```python
from build123d import *

# Parameters (mm, degrees)
F1_DEPTH  = 15.875
F3_DEPTH  = 15.876
F4_R      = 15.1511
F5_DEPTH  = 15.876
F6_R      = 57.277
F7_DEPTH  = 6.35
F8_R      = 4.953
F9_DEPTH  = 15.876
F11_DEPTH = 9.525
F13_R     = 5.4864
F14_DEPTH = 15.875
F16_DEPTH = 1.27


with BuildPart() as f1:
    # F0 (on Top) → F1 (new body)
    with BuildSketch(Plane.XY):
        with BuildLine():
            Line((261.564905, -58.477244), (113.604486, -6.008632))
            ThreePointArc((113.604486, -6.008632), (0, -82.6643), (113.604486, -159.319968))
            Line((113.604486, -159.319968), (261.564905, -106.851356))
            Line((261.564905, -106.851356), (263.024603, -106.333729))
            ThreePointArc((263.024603, -106.333729), (279.2095, -82.6643), (263.024603, -58.994871))
            Line((263.024603, -58.994871), (261.564905, -58.477244))
        make_face()
        with BuildLine():
            ThreePointArc((263.024603, -58.994871), (262.2987, -58.724929), (261.564905, -58.477244))
            Line((261.564905, -58.477244), (263.024603, -58.994871))
        make_face()
        with BuildLine():
            Line((263.024603, -106.333729), (261.564905, -106.851356))
            ThreePointArc((261.564905, -106.851356), (262.2987, -106.603671), (263.024603, -106.333729))
        make_face()
    extrude(amount=F1_DEPTH)

    # F2 (on face) → F3 (cut, through all)
    with BuildSketch(Plane.XY.offset(15.875)):
        with BuildLine():
            ThreePointArc((266.5095, -82.6643), (253.8095, -69.9643), (241.1095, -82.6643))
            Line((241.1095, -82.6643), (266.5095, -82.6643))
        make_face()
        with BuildLine():
            Line((266.5095, -82.6643), (241.1095, -82.6643))
            ThreePointArc((241.1095, -82.6643), (253.8095, -95.3643), (266.5095, -82.6643))
        make_face()
    extrude(amount=-F3_DEPTH, mode=Mode.SUBTRACT)

    # F4 (on face) → F5 (cut, through all)
    with BuildSketch(Plane.XY.offset(15.875)):
        with Locations((82.3595, -82.6643)):
            Circle(F4_R)
    extrude(amount=-F5_DEPTH, mode=Mode.SUBTRACT)

    # F6 (on face) → F7 (cut)
    with BuildSketch(Plane(origin=(0, 0, 0), x_dir=(1, 0, 0), z_dir=(0, 0, -1))):
        with Locations((82.3595, 82.6643)):
            Circle(F6_R)
    extrude(amount=-F7_DEPTH, mode=Mode.SUBTRACT)

    # F8 (on face) → F9 (cut, through all)
    with BuildSketch(Plane(origin=(0, 0, 0), x_dir=(1, 0, 0), z_dir=(0, 0, -1))):
        with Locations((29.6545, 135.3693)):
            Circle(F8_R)
        with Locations((135.0645, 135.3693)):
            Circle(F8_R)
        with Locations((135.0645, 29.9593)):
            Circle(F8_R)
        with Locations((29.6545, 29.9593)):
            Circle(F8_R)
    extrude(amount=-F9_DEPTH, mode=Mode.SUBTRACT)

    # F10 (on face) → F11 (cut)
    with BuildSketch(Plane(origin=(0, 0, 0), x_dir=(1, 0, 0), z_dir=(0, 0, -1))):
        with BuildLine():
            ThreePointArc((57.15, 82.6643), (56.220064, 84.909364), (53.975, 85.8393))
            Line((53.975, 85.8393), (0.060996, 85.8393))
            Line((0.060996, 85.8393), (-2.488084, 85.8393))
            Line((-2.488084, 85.8393), (-2.488084, 79.4893))
            Line((-2.488084, 79.4893), (-1.513804, 79.4893))
            Line((-1.513804, 79.4893), (53.975, 79.4893))
            ThreePointArc((53.975, 79.4893), (56.220064, 80.419236), (57.15, 82.6643))
        make_face()
    extrude(amount=-F11_DEPTH, mode=Mode.SUBTRACT)

    # F13 (on offset) → F14 (cut)
    with BuildSketch(Plane.YZ.offset(279.4)):
        with Locations((-82.6643, 7.9375)):
            Circle(F13_R)
    extrude(amount=-F14_DEPTH, mode=Mode.SUBTRACT)

    # F15 (on face) → F16 (cut)
    with BuildSketch(Plane.XY.offset(15.875)):
        with BuildLine():
            Line((167.299575, -48.660433), (144.385987, -48.660433))
            Line((144.385987, -48.660433), (148.052161, -55.010433))
            Line((148.052161, -55.010433), (172.798837, -55.010433))
            ThreePointArc((172.798837, -55.010433), (173.592587, -55.223117), (174.173652, -55.804183))
            Line((174.173652, -55.804183), (207.672688, -113.826216))
            Line((207.672688, -113.826216), (214.81237, -113.492506))
            Line((214.81237, -113.492506), (172.90237, -40.902257))
            Line((172.90237, -40.902257), (165.468663, -40.726699))
            Line((165.468663, -40.726699), (168.674391, -46.279183))
            ThreePointArc((168.674391, -46.279183), (168.674391, -47.866683), (167.299575, -48.660433))
        make_face()
        with BuildLine():
            Line((165.826053, -66.122933), (171.684878, -66.122933))
            Line((171.684878, -66.122933), (175.980346, -73.562901))
            Line((175.980346, -73.562901), (177.355162, -72.769151))
            Line((177.355162, -72.769151), (178.729977, -71.975401))
            Line((178.729977, -71.975401), (174.434509, -64.535433))
            ThreePointArc((174.434509, -64.535433), (173.272378, -63.373302), (171.684878, -62.947933))
            Line((171.684878, -62.947933), (156.301053, -62.947933))
            ThreePointArc((156.301053, -62.947933), (153.551422, -64.535433), (153.551422, -67.710433))
            Line((153.551422, -67.710433), (156.930346, -73.562901))
            Line((156.930346, -73.562901), (158.305162, -72.769151))
            Line((158.305162, -72.769151), (159.679977, -71.975401))
            Line((159.679977, -71.975401), (156.301053, -66.122933))
            Line((156.301053, -66.122933), (162.159878, -66.122933))
            Line((162.159878, -66.122933), (165.095358, -71.207332))
            Line((165.095358, -71.207332), (167.844988, -69.619832))
            Line((167.844988, -69.619832), (165.826053, -66.122933))
        make_face()
        with BuildLine():
            Line((166.832487, -84.363913), (162.863737, -77.489836))
            Line((162.863737, -77.489836), (160.114107, -79.077336))
            Line((160.114107, -79.077336), (164.082857, -85.951413))
            ThreePointArc((164.082857, -85.951413), (166.010737, -87.430727), (168.419987, -87.113543))
            Line((168.419987, -87.113543), (179.957857, -80.452151))
            Line((179.957857, -80.452151), (183.926607, -87.326228))
            Line((183.926607, -87.326228), (186.676237, -85.738728))
            Line((186.676237, -85.738728), (182.707487, -78.864651))
            ThreePointArc((182.707487, -78.864651), (180.779607, -77.385337), (178.370357, -77.702521))
            Line((178.370357, -77.702521), (166.832487, -84.363913))
        make_face()
        with BuildLine():
            Line((172.176053, -93.619239), (187.559878, -93.619239))
            Line((187.559878, -93.619239), (191.864107, -101.074381))
            Line((191.864107, -101.074381), (194.613737, -99.486881))
            Line((194.613737, -99.486881), (190.309509, -92.031739))
            ThreePointArc((190.309509, -92.031739), (189.147378, -90.869609), (187.559878, -90.444239))
            Line((187.559878, -90.444239), (172.176053, -90.444239))
            ThreePointArc((172.176053, -90.444239), (169.426422, -92.031739), (169.426422, -95.206739))
            Line((169.426422, -95.206739), (172.814107, -101.074381))
            Line((172.814107, -101.074381), (175.563737, -99.486881))
            Line((175.563737, -99.486881), (172.176053, -93.619239))
        make_face()
        with BuildLine():
            Line((201.252318, -110.681192), (198.234108, -105.717761))
            ThreePointArc((198.234108, -105.717761), (197.077421, -104.599884), (195.521297, -104.192393))
            Line((195.521297, -104.192393), (180.187231, -104.192393))
            ThreePointArc((180.187231, -104.192393), (177.419723, -105.811268), (177.474421, -109.017024))
            Line((177.474421, -109.017024), (180.492631, -113.980455))
            ThreePointArc((180.492631, -113.980455), (181.649318, -115.098332), (183.205442, -115.505824))
            Line((183.205442, -115.505824), (198.539508, -115.505824))
            ThreePointArc((198.539508, -115.505824), (201.307016, -113.886948), (201.252318, -110.681192))
        make_face()
        Polygon((183.205442, -112.330824), (180.187231, -107.367393), (195.521297, -107.367393), (198.539508, -112.330824), align=None, mode=Mode.SUBTRACT)
    extrude(amount=-F16_DEPTH, mode=Mode.SUBTRACT)


solid = f1.part
```
Check sheet for the modelled part. Datum: model origin and axes. Units: mm. A direction names the side the tool comes from. Round coordinates to 2 decimals unless told otherwise and drop trailing zeros. Order: outer loops, then holes, each group sorted by start corner. A loop starts at its lowest first (then second) coordinate and runs counter-clockwise, first axis right, second up. Notation, with made-up numbers: (38.25, -25.5) - (80.25, -25.5) arc R21 ccw to (80.25, -9.5) - close; hole circle Ø1 at (61, 81). An arc over 180 degrees is marked (long way). Write item = value, one per line.
Q1. Section check B-B (x = 205). Record the boundary of the cut face in (y, z) (3 decimals).
Computed:
outline = (-126.91, 0) - (-38.419, 0) - (-38.419, 15.875) - (-96.497, 15.875) - (-96.497, 14.605) - (-109.197, 14.605) - (-109.197, 15.875) - (-126.91, 15.875) - close
Q2. Section check A-A (x = 249). Record the boundary of the cut face in (y, z) (3 decimals), and give its area (3 significant figures).
Computed:
outline = (-111.307, 0) - (-94.418, 0) - (-94.418, 15.875) - (-111.307, 15.875) - close; (-70.91, 0) - (-54.022, 0) - (-54.022, 15.875) - (-70.91, 15.875) - close
area = 536 mm^2
Q3. Thickness scan on line 1 along X through (y, z) = (-94, 3.75); line 2 along X through (y, z) = (-72, 15.25); line 3 along X through (y, z) = (-73.5, 7.5). Record the ranges inside material, lowest first.
Computed:
line_1 = 0.78 to 26.22, 138.5 to 248.08, 259.54 to 276.54
line_2 = 0.69 to 71.6, 93.12 to 156.03, 159.64 to 175.08, 178.69 to 183.52, 190.86 to 246.91, 260.71 to 276.86
line_3 = 0.51 to 70.29, 94.42 to 245.02, 262.6 to 277.5
Q4. Go/stop test with flat-tipped pins: pin 1 (1 mm diameter, centred on x = 174, y = -100, fed in from -Z); pin 2 (6 mm diameter, centred on x = 135.06, y = -29.96, fed in from +Z); pin 3 (1.4 mm diameter, centred on x = 189.5, z = 15, fed in from -Y); pin 4 (0.6 mm diameter, centred on x = 188, z = 15, fed in from +Y). Record where each tip stops, or that it passes through.
Computed:
pin_1 = 0
pin_2 = through
pin_3 = -132.65
pin_4 = -32.28
Q5. Tool access check on faces 1 (the face through (188.62, -32.61, 7.83)), 2 (the face through (173, -82, 14.605)), 3 (the face through (24.706, -30.177, 7.826)), 4 (the face through (94, -71, 6.35)), 5 (the face through (21, -85.839, 6)). Record the directions out of +Z, -Z, +X, -X, +Y, -Y that give a thin tool (end or side, any length) a straight path to the whole face; none if there is none.
Computed:
face_1 = +Z, -Z, +X, +Y
face_2 = +Z
face_3 = +Z, -Z
face_4 = -Z
face_5 = -Z, -X
Q6. Section check C-C (x = 73). Record the boundary of the cut face in (y, z) (3 decimals).
Computed:
outline = (-164.762, 0) - (-139.171, 0) - (-139.171, 6.35) - (-94.579, 6.35) - (-94.579, 15.875) - (-164.762, 15.875) - close; (-70.75, 6.35) - (-26.157, 6.35) - (-26.157, 0) - (-0.567, 0) - (-0.567, 15.875) - (-70.75, 15.875) - close
Q7. Section check D-D (y = -150.5). Record the boundary of the cut face in (x, z) (3 decimals).
Computed:
outline = (35.423, 0) - (138.477, 0) - (138.477, 15.875) - (35.423, 15.875) - close
